Could you check a few things on this drawing? It's one solid part, dimensions in mm from its lowest x, y, z. Round coordinates to 2 decimals unless told otherwise and drop trailing zeros. Loops run counter-clockwise (first coordinate to the right, second up) from the corner with the lowest first, then second, coordinate; pieces in that order, holes last. Notation, with made-up numbers: (32.5, 23.25) -> (65.5, 23.25) arc R26 ccw to (65.5, 49.25) -> close; hole circle Ø10 at (10, 70). An arc over 180 degrees is marked (long way). Use one line per item in the form item = value. Start each with the question number.
Item 1: If we section it at C-C (z = 8): Write out the boundary of the cut face in (x, y) (1 decimal).
Item 2: If I drill on L1, parallel to X at y = 23, z = 16.25 (1 decimal); L2, parallel to Y at x = 3.5, z = 20.25 (1 decimal); L3, parallel to Z at x = 14, y = 31, over which ranges is the centre line in solid material (lowest first)? Write a range as [from, to].
Item 3: Thinking about a two-plate mould opening in Z: for the marked faces 1, 2 and 3, which applies, released by +Z, released by -Z, zero draft, split by the parting line, or undercut?
Item 4: I'm going to push flat-ended pins straight in: pin 1 Ø1 at (x, z) = (12, 18.5) entering from -Y; pin 2 Ø12 at (x, z) = (5, 11.5) entering from -Y; pin 3 Ø5 at (y, z) = (26.5, 3) entering from -X (1 decimal). Where does each tip first touch, or does it pass through?
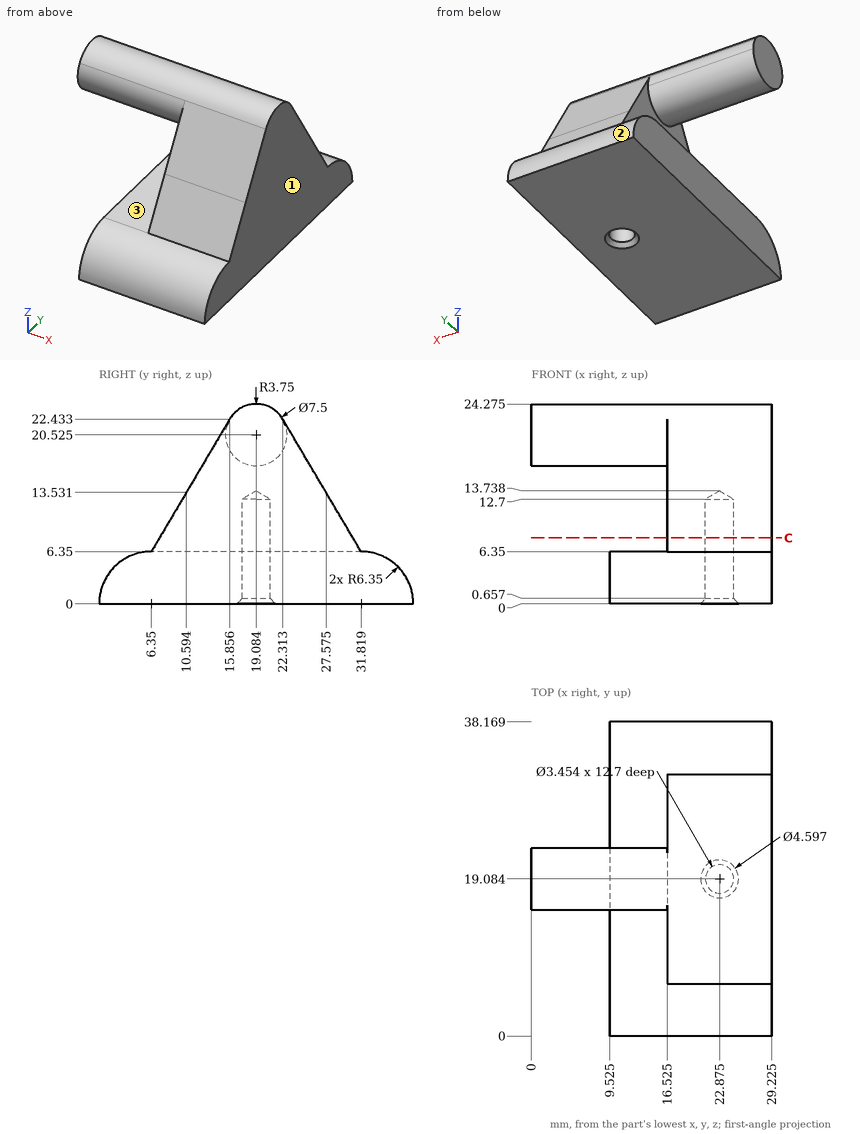
Values found:
q1.outline = (16.5, 7.3) -> (29.2, 7.3) -> (29.2, 30.8) -> (16.5, 30.8) -> close; hole circle Ø3.5 at (22.9, 19.1)
q2.L1 = [16.5, 29.2]
q2.L2 = [15.3, 22.8]
q2.L3 = [0, 6.35]
q3.face_1 = zero draft
q3.face_2 = released by +Z
q3.face_3 = undercut
q4.pin_1 = 15.66
q4.pin_2 = 16.87
q4.pin_3 = 9.5
